```python
from build123d import *

# Parameters (mm, degrees)
CROQUIS1_W              = 50
CROQUIS1_H              = 50
CROQUIS1_R              = 1.35
SALIENTE_EXTRUIR1_DEPTH = 24
CROQUIS2_R              = 7.5
SALIENTE_EXTRUIR2_DEPTH = 40


with BuildPart() as part:
    # Croquis1 → Saliente-Extruir1 (new body)
    with BuildSketch(Plane(origin=(0, 0, 0), x_dir=(1, 0, 0), z_dir=(0, 1, 0))):
        Rectangle(CROQUIS1_W, CROQUIS1_H)
        with Locations(Location((-15, 15, 0), (0, 0, 270))):
            Circle(CROQUIS1_R, mode=Mode.SUBTRACT)
        with Locations(Location((15, 15, 0), (0, 0, 90))):
            Circle(CROQUIS1_R, mode=Mode.SUBTRACT)
        with Locations(Location((-15, -15, 0), (0, 0, 90))):
            Circle(CROQUIS1_R, mode=Mode.SUBTRACT)
        with Locations(Location((15, -15, 0), (0, 0, 270))):
            Circle(CROQUIS1_R, mode=Mode.SUBTRACT)
    extrude(amount=SALIENTE_EXTRUIR1_DEPTH)

    # Croquis2 → Saliente-Extruir2 (add)
    with BuildSketch(Plane(origin=(0, 0, 0), x_dir=(1, 0, 0), z_dir=(0, 1, 0))):
        with Locations(Location((0, 0, 0), (0, 0, 90))):
            Circle(CROQUIS2_R)
    extrude(amount=SALIENTE_EXTRUIR2_DEPTH)

    # Croquis3 → Revolución1 (revolve)
    with BuildSketch(Plane(origin=(0, 55, 0), x_dir=(1, 0, 0), z_dir=(0, 1, 0))):
        with BuildLine():
            Line((0, 16.5), (0, -16.5))
            ThreePointArc((0, -16.5), (16.5, 0), (0, 16.5))
        make_face()
    revolve(axis=Axis((0, 55, -16.5), (0, 0, 1)))


solid = part.part
```
Design review of the part built by this model. Coordinates are the model's own, in mm. A direction names the side the tool comes from. Coordinates: 2 decimals unless noted, no trailing zeros. Order: outer loops, then holes, each group sorted by start corner. A loop starts at its lowest first (then second) coordinate and runs counter-clockwise, first axis right, second up.
1) For faces 1 (the flat face through (2, 40, -7)), 2 (the cylindrical face through (-13.661, 11.832, -15.176)), list the 3-axis set-ups (+Z, -Z, +X, -X, +Y, -Y) from which the entire face can be reached by the end or side of a thin tool; tool diameter is ignored.
2) Take a section at A-A, the plane x = 15. Give the boundary of the cut face in (y, z).
3) Take a section at B-B, the plane z = -14.5. Give the boundary of the cut face in (x, y), and give its area (3 significant figures).
4) Take a section at D-D, the plane x = -4.5. Give the boundary of the cut face in (y, z).
5) Mouldability with a two-part tool opening along Y and no side actions: class faces 3 (the flat face through (0, 0, 0)), 4 (the flat face through (-6, 24, -6)), 5 (the flat face through (-25, 12, 0)), 6 (the cylindrical face through (-0.33, 31.888, 7.493)) as +Y half, -Y half, draft (parallel to the pull), parting line (faces both ways), or undercut.
6) Take a section at C-C, the plane z = -1.5. Give the boundary of the cut face in (x, y), and give its area (3 significant figures).
7) Wall thickness on line 1 along X through (y, z) = (11.25, -15); line 2 along Y through (x, z) = (14.5, -8.5); line 3 along Y through (x, z) = (-9, 3): over which ranges is each line inside the solid? List them lowest first.
8) Clearance check with flat-ended pins moving along their axes: pin 1 (3 mm diameter, centred on x = 4, y = 46.5, fed in from +Z); pin 2 (6 mm diameter, centred on y = 42.5, z = 3, fed in from +X); pin 3 (1 mm diameter, centred on x = 7, y = 59, fed in from -Z) (3 decimals). State where each tip first meets the part, or that it passes through.
Returned:
1. face 1: none
1. face 2: +Y, -Y
2. outline: (0, -25) - (24, -25) - (24, -16.35) - (0, -16.35) - close; (0, -13.65) - (24, -13.65) - (24, 13.65) - (0, 13.65) - close; (0, 16.35) - (24, 16.35) - (24, 25) - (0, 25) - close; circle Ø13.75 at (55, 0)
3. outline: (-25, 0) - (-16.25, 0) - (-16.25, 24) - (-25, 24) - close; (-13.75, 0) - (13.75, 0) - (13.75, 24) - (-13.75, 24) - close; circle Ø15.75 at (0, 55); (16.25, 0) - (25, 0) - (25, 24) - (16.25, 24) - close
3. area: 1,270 mm2
4. outline: (0, -25) - (24, -25) - (24, -6) - (40, -6) - (40, -5.2) arc R15.87 ccw (long way) to (40, 5.2) - (40, 6) - (24, 6) - (24, 25) - (0, 25) - close
5. face 3: -Y half
5. face 4: undercut
5. face 5: draft
5. face 6: undercut
6. outline: (-25, 0) - (25, 0) - (25, 24) - (7.35, 24) - (7.35, 40) - (6.71, 40) arc R16.43 ccw (long way) to (-6.71, 40) - (-7.35, 40) - (-7.35, 24) - (-25, 24) - close
6. area: 2,270 mm2
7. line 1: x = -25 to -16.35, -13.65 to 13.65, 16.35 to 25
7. line 2: y = 0 to 24
7. line 3: y = 0 to 24, 41.5 to 68.5
8. pin 1: stops at z = 14.49
8. pin 2: stops at x = 13.23
8. pin 3: stops at z = -14.665
